from build123d import *

# Parameters (mm, degrees)
CROQUIS2_R                        = 21
CROQUIS2_R_2                      = 8.05
SALIENTE_EXTRUIR1_DEPTH           = 4
CROQUIS3_R                        = 12.05
CROQUIS3_R_2                      = 8.05
SALIENTE_EXTRUIR2_DEPTH           = 8
REDONDEO1_R                       = 4
CORTAR_EXTRUIR2_REACH             = 34.031
CROQUIS5_R                        = 4.05
CROQUIS4_R                        = 1.625
CORTAR_EXTRUIR3_DEPTH             = 33.031234794
CORTAR_EXTRUIR4_REACH             = 41.705
CROQUIS6_R                        = 1.625
CORTAR_EXTRUIR4_DIRECTION_2_REACH = 41.705
CROQUIS7_R                        = 4.05
CROQUIS7_R_2                      = 3.05
SALIENTE_EXTRUIR3_DEPTH           = 1
CHAFL_N1_SIZE                     = 0.5
CORTAR_EXTRUIR5_REACH             = 41.705
CROQUIS8_R                        = 1.625
CORTAR_EXTRUIR5_DIRECTION_2_REACH = 41.705


with BuildPart() as part:
    # Croquis2 → Saliente-Extruir1 (new body)
    with BuildSketch(Plane(origin=(0, 0, 0), x_dir=(1, 0, 0), z_dir=(0, 1, 0))):
        with Locations(Location((0, 0, 0), (0, 0, 270))):
            Circle(CROQUIS2_R)
        with Locations(Location((0, 0, 0), (0, 0, 270))):
            Circle(CROQUIS2_R_2, mode=Mode.SUBTRACT)
    extrude(amount=SALIENTE_EXTRUIR1_DEPTH)

    # Croquis3 → Saliente-Extruir2 (add)
    with BuildSketch(Plane(origin=(0, 4, 0), x_dir=(1, 0, 0), z_dir=(0, 1, 0))):
        with Locations(Location((0, 0, 0), (0, 0, 270))):
            Circle(CROQUIS3_R)
        with Locations(Location((0, 0, 0), (0, 0, 270))):
            Circle(CROQUIS3_R_2, mode=Mode.SUBTRACT)
    extrude(amount=SALIENTE_EXTRUIR2_DEPTH)

    # Redondeo1
    redondeo1_edges = [part.edges().sort_by_distance(p)[0] for p in [
        (0, 4, -12.05),
    ]]
    fillet(redondeo1_edges, radius=REDONDEO1_R)

    # Croquis5 → Cortar-Extruir2 (cut, up to next)
    with BuildSketch(Plane.XZ, mode=Mode.PRIVATE) as cortar_extruir2_sk1:
        with Locations(Location((0, 14.5, 0), (0, 0, 270))):
            Circle(CROQUIS5_R)
    cortar_extruir2_tool1 = extrude(cortar_extruir2_sk1.sketch, amount=-CORTAR_EXTRUIR2_REACH, mode=Mode.PRIVATE) & part.part
    # Croquis5 → Cortar-Extruir2 (cut, up to next)
    with BuildSketch(Plane.XZ, mode=Mode.PRIVATE) as cortar_extruir2_sk2:
        with Locations(Location((12.557368355, -7.25, 0), (0, 0, 270))):
            Circle(CROQUIS5_R)
    cortar_extruir2_tool2 = extrude(cortar_extruir2_sk2.sketch, amount=-CORTAR_EXTRUIR2_REACH, mode=Mode.PRIVATE) & part.part
    # Croquis5 → Cortar-Extruir2 (cut, up to next)
    with BuildSketch(Plane.XZ, mode=Mode.PRIVATE) as cortar_extruir2_sk3:
        with Locations(Location((-12.557368355, -7.25, 0), (0, 0, 270))):
            Circle(CROQUIS5_R)
    cortar_extruir2_tool3 = extrude(cortar_extruir2_sk3.sketch, amount=-CORTAR_EXTRUIR2_REACH, mode=Mode.PRIVATE) & part.part
    add(cortar_extruir2_tool1.solids().sort_by_distance((0, 0, 14.5))[0], mode=Mode.SUBTRACT)
    add(cortar_extruir2_tool2.solids().sort_by_distance((12.557368, 0, -7.25))[0], mode=Mode.SUBTRACT)
    add(cortar_extruir2_tool3.solids().sort_by_distance((-12.557368, 0, -7.25))[0], mode=Mode.SUBTRACT)

    # Croquis4 → Cortar-Extruir3 (cut, through all)
    with BuildSketch(Plane.XY):
        with Locations((0, 8)):
            Circle(CROQUIS4_R)
    extrude(amount=-CORTAR_EXTRUIR3_DEPTH, mode=Mode.SUBTRACT)

    # Croquis6 → Cortar-Extruir4 (cut, up to next)
    with BuildSketch(Plane(origin=(7.250941954, 0, 4.186333289), x_dir=(-0.5000000000000033, 0, 0.8660254037844367), z_dir=(-0.8660254037844367, 0, -0.5000000000000033)), mode=Mode.PRIVATE) as cortar_extruir4_sk1:
        with Locations(Location((0, 8, 0), (0, 0, 180))):
            Circle(CROQUIS6_R)
    cortar_extruir4_tool1 = extrude(cortar_extruir4_sk1.sketch, amount=-CORTAR_EXTRUIR4_REACH, mode=Mode.PRIVATE) & part.part
    add(cortar_extruir4_tool1.solids().sort_by_distance((7.250942, 8, 4.186333))[0], mode=Mode.SUBTRACT)

    # Croquis6 → Cortar-Extruir4 direction 2 (cut, up to next)
    with BuildSketch(Plane(origin=(7.250941954, 0, 4.186333289), x_dir=(-0.5000000000000033, 0, 0.8660254037844367), z_dir=(-0.8660254037844367, 0, -0.5000000000000033)), mode=Mode.PRIVATE) as cortar_extruir4_direction_2_sk1:
        with Locations(Location((0, 8, 0), (0, 0, 180))):
            Circle(CROQUIS6_R)
    cortar_extruir4_direction_2_tool1 = extrude(cortar_extruir4_direction_2_sk1.sketch, amount=CORTAR_EXTRUIR4_DIRECTION_2_REACH, mode=Mode.PRIVATE) & part.part
    add(cortar_extruir4_direction_2_tool1.solids().sort_by_distance((7.250942, 8, 4.186333))[0], mode=Mode.SUBTRACT)

    # Croquis7 → Saliente-Extruir3 (add)
    # profile 1 of 3: a face of its own
    with BuildSketch(Plane.XZ):
        with Locations(Location((0, 14.5, 0), (0, 0, 270))):
            Circle(CROQUIS7_R)
        with Locations(Location((0, 14.5, 0), (0, 0, 270))):
            Circle(CROQUIS7_R_2, mode=Mode.SUBTRACT)
    # profile 2 of 3: a face of its own
    with BuildSketch(Plane.XZ):
        with Locations(Location((12.557368355, -7.25, 0), (0, 0, 270))):
            Circle(CROQUIS7_R)
        with Locations(Location((12.557368355, -7.25, 0), (0, 0, 270))):
            Circle(CROQUIS7_R_2, mode=Mode.SUBTRACT)
    # profile 3 of 3: a face of its own
    with BuildSketch(Plane.XZ):
        with Locations(Location((-12.557368355, -7.25, 0), (0, 0, 270))):
            Circle(CROQUIS7_R)
        with Locations(Location((-12.557368355, -7.25, 0), (0, 0, 270))):
            Circle(CROQUIS7_R_2, mode=Mode.SUBTRACT)
    extrude(amount=-SALIENTE_EXTRUIR3_DEPTH)

    # Chaflán1
    chafl_n1_edges = [part.edges().sort_by_distance(p)[0] for p in [
        (0, 12, -8.05),
        (0, 0, -8.05),
    ]]
    chamfer(chafl_n1_edges, length=CHAFL_N1_SIZE)

    # Croquis8 → Cortar-Extruir5 (cut, up to next)
    with BuildSketch(Plane(origin=(-7.250941954, 0, 4.186333289), x_dir=(-0.5000000000000002, 0, -0.8660254037844386), z_dir=(0.8660254037844386, 0, -0.5000000000000002)), mode=Mode.PRIVATE) as cortar_extruir5_sk1:
        with Locations(Location((0, 8, 0), (0, 0, 180))):
            Circle(CROQUIS8_R)
    cortar_extruir5_tool1 = extrude(cortar_extruir5_sk1.sketch, amount=-CORTAR_EXTRUIR5_REACH, mode=Mode.PRIVATE) & part.part
    add(cortar_extruir5_tool1.solids().sort_by_distance((-7.250942, 8, 4.186333))[0], mode=Mode.SUBTRACT)

    # Croquis8 → Cortar-Extruir5 direction 2 (cut, up to next)
    with BuildSketch(Plane(origin=(-7.250941954, 0, 4.186333289), x_dir=(-0.5000000000000002, 0, -0.8660254037844386), z_dir=(0.8660254037844386, 0, -0.5000000000000002)), mode=Mode.PRIVATE) as cortar_extruir5_direction_2_sk1:
        with Locations(Location((0, 8, 0), (0, 0, 180))):
            Circle(CROQUIS8_R)
    cortar_extruir5_direction_2_tool1 = extrude(cortar_extruir5_direction_2_sk1.sketch, amount=CORTAR_EXTRUIR5_DIRECTION_2_REACH, mode=Mode.PRIVATE) & part.part
    add(cortar_extruir5_direction_2_tool1.solids().sort_by_distance((-7.250942, 8, 4.186333))[0], mode=Mode.SUBTRACT)


solid = part.part
The model under review builds one solid part; all positions refer to its coordinate system, in mm. A direction names the side the tool comes from. Give positions to 0.01 mm unless a question says otherwise; leave off trailing zeros. Loops run counter-clockwise (first coordinate to the right, second up) from the corner with the lowest first, then second, coordinate; pieces in that order, holes last. Notation, with made-up numbers: (34.5, 49.25) -> (53.5, 49.25) arc R28 ccw to (53.5, 70.25) -> close; hole circle Ø2 at (59, 84.25). An arc over 180 degrees is marked (long way). Answer as a JSON object with one key per item and string values. Group by question number.
Q1. Insertion check: pin 1 (2 mm diameter, centred on x = 13.5, z = -7.5, fed in from +Y); pin 2 (2.5 mm diameter, centred on x = 0.5, z = 16.5, fed in from +Y); pin 3 (3.5 mm diameter, centred on x = 0, y = 8, fed in from +Z); pin 4 (5 mm diameter, centred on y = 10, z = -7, fed in from -X). Each pin has a flat end and moves straight along its axis. Give the tip position at first contact, or say it passes through.
Q2. Tool access review of faces 5 (the cylindrical face through (8.65, 6.39, 5.24)), 6 (the flat face through (-9.5, 1, -6.3)): name each direction out of +Z, -Z, +X, -X, +Y, -Y from which nothing blocks a thin tool from reaching the whole face with its end or side.
Q3. Take a section at B-B (x = 0). Write out the cut boundary in (y, z) (3 decimals).
Q4. Draft analysis for pull direction X (two halves, no side actions). For faces 1 (the flat face through (-9, 0, 0)), 2 (the cylindrical face through (0.75, 6.56, -10.11)), 3 (the cylindrical face through (0.14, 9.97, -12.05)), 4 (the cylindrical face through (10.37, 9.97, 6.14)), state which applies: pulls with the +X half, pulls with the -X half, needs draft (parallel to the pull), parting line crosses it, or undercut.
Q5. Take a section at A-A (z = 0). Write out the cut boundary in (x, y).
Q6. Wall thickness on line 1 along X through (y, z) = (3.75, 0); line 2 along X through (y, z) = (0.3, -7.25); line 3 along X through (y, z) = (2, -6): over which ranges is each line inside the solid? List them lowest first.
Q7. Take a section at D-D (z = -7.25). State how many separate pieces and enclosed holes the cut face has, plus the area to 3 significant figures.
Answer below:
{
 "1": {"pin 1": "passes through", "pin 2": "stops at y = 1", "pin 3": "stops at z = 10.85", "pin 4": "stops at x = -9.58"},
 "2": {"face 5": "none", "face 6": "+Y"},
 "3": {"outline": "(0, -21) -> (4, -21) -> (4, -16.05) arc R4 cw to (6.375, -12.395) -> (6.375, -8.05) -> (0.5, -8.05) -> (0, -8.55) -> close; (0, 8.55) -> (0.5, 8.05) -> (11.5, 8.05) -> (12, 8.55) -> (12, 10.45) -> (1, 10.45) -> (1, 11.45) -> (0, 11.45) -> close; (0, 17.55) -> (1, 17.55) -> (1, 18.55) -> (4, 18.55) -> (4, 21) -> (0, 21) -> close; (9.625, -12.05) -> (12, -12.05) -> (12, -8.55) -> (11.5, -8.05) -> (9.625, -8.05) -> close"},
 "4": {"face 1": "needs draft", "face 2": "undercut", "face 3": "parting line crosses it", "face 4": "pulls with the +X half"},
 "5": {"outline": "(-21, 0) -> (-8.55, 0) -> (-8.05, 0.5) -> (-8.05, 11.5) -> (-8.55, 12) -> (-12.05, 12) -> (-12.05, 8) arc R4 cw to (-16.05, 4) -> (-21, 4) -> close; (8.05, 0.5) -> (8.55, 0) -> (21, 0) -> (21, 4) -> (16.05, 4) arc R4 cw to (12.05, 8) -> (12.05, 12) -> (8.55, 12) -> (8.05, 11.5) -> close"},
 "6": {"line 1": "x = -21 to -8.05, 8.05 to 21", "line 2": "x = -19.71 to -15.61, -9.51 to -3.94, 3.94 to 9.51, 15.61 to 19.71", "line 3": "x = -20.12 to -16.41, -8.71 to -5.37, 5.37 to 8.71, 16.41 to 20.12"},
 "7": {"separate pieces": "4", "enclosed holes": "0", "area": "148 mm2"}
}
